Geometry check sheet. Reference: the model listing, model coordinates, mm. Face numbers are marked on the shaded views. A direction names the side the tool comes from. Round coordinates to 2 decimals unless told otherwise and drop trailing zeros. Write each loop counter-clockwise with the first axis right and the second up, starting at its lowest first coordinate (ties: lowest second). Pieces come first, ordered by that corner, then holes. Notation, with made-up numbers: (-17, -22.75) -> (0, -22.75) arc R11 ccw to (0, -4.75) -> close; hole circle Ø7 at (47, 38). An arc over 180 degrees is marked (long way). Use a Markdown table: item, result.
```python
from build123d import *

# Parameters (mm, degrees)
SKETCH1_R               = 13.85
BOSS_EXTRUDE1_DEPTH     = 63
CUT_EXTRUDE1_DEPTH      = 66.974578437
CUT_EXTRUDE1_DEPTH_BACK = 66.974578437


with BuildPart() as part:
    # Sketch1 → Boss-Extrude1 (new body)
    with BuildSketch(Plane.XY):
        Circle(SKETCH1_R)
    extrude(amount=BOSS_EXTRUDE1_DEPTH)

    # Sketch3 → Cut-Extrude1 (cut, two sides: drawn at the far end of the back side and taken through both)
    with BuildSketch(Plane(origin=(0, 0, 0), x_dir=(0, 0, -1), z_dir=(1, 0, 0)).offset(-CUT_EXTRUDE1_DEPTH_BACK)):
        with BuildLine():
            Line((0, 1.925), (-35.5, 1.925))
            ThreePointArc((-35.5, 1.925), (-37.267766953, 2.657233047), (-38, 4.425))
            Line((-38, 4.425), (-38, 13.85))
            Line((-38, 13.85), (0, 13.85))
            Line((0, 13.85), (0, 1.925))
        make_face()
        with BuildLine():
            Line((0, -1.925), (-45.5, -1.925))
            ThreePointArc((-45.5, -1.925), (-47.267766953, -2.657233047), (-48, -4.425))
            Line((-48, -4.425), (-48, -13.85))
            Line((-48, -13.85), (0, -13.85))
            Line((0, -13.85), (0, -1.925))
        make_face()
    extrude(amount=CUT_EXTRUDE1_DEPTH + CUT_EXTRUDE1_DEPTH_BACK, mode=Mode.SUBTRACT)


solid = part.part
```
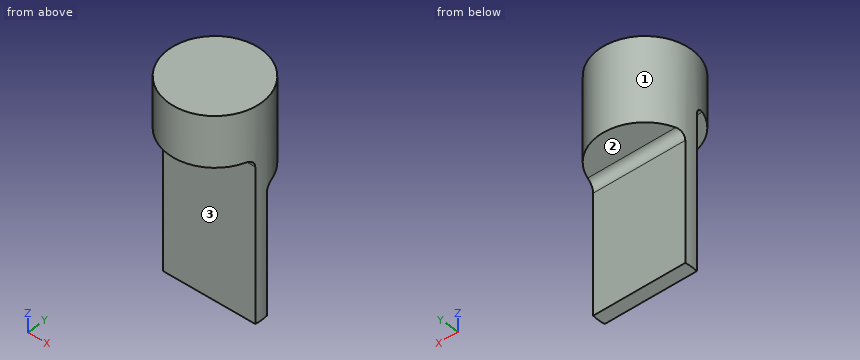
(1) Section check D-D on x = -9.75. Record the cut outline in (y, z) (3 decimals), plus the area to 3 significant figures.
A:
| item | result |
|---|---|
| outline | (-9.837, 48) -> (-4.425, 48) arc R2.5 cw to (-1.925, 45.5) -> (-1.925, 0) -> (1.925, 0) -> (1.925, 35.5) arc R2.5 cw to (4.425, 38) -> (9.837, 38) -> (9.837, 63) -> (-9.837, 63) -> close |
| area | 562 mm2 |
(2) Section check B-B on z = 27.5. Record the cut outline in (x, y) (3 decimals), plus the area to 3 significant figures.
A:
| item | result |
|---|---|
| outline | (-13.716, -1.925) -> (13.716, -1.925) arc R13.85 ccw to (13.716, 1.925) -> (-13.716, 1.925) arc R13.85 ccw to start |
| area | 106 mm2 |
(3) Thickness scan on line 1 (Y direction, x = 6, z = 30) (3 decimals); line 2 (Z direction, x = 3.25, y = 6.5); line 3 (Z direction, x = -6.75, y = -4.5). Record the ranges inside material, lowest first.
A:
| item | result |
|---|---|
| line 1 | y = -1.925 to 1.925 |
| line 2 | z = 38 to 63 |
| line 3 | z = 48 to 63 |
(4) Access from +Z, -Z, +X, -X, +Y, -Y to the whole of each face (thin tool, end or side, straight path). Record for the marked faces 1, 2 and 3.
A:
| item | result |
|---|---|
| face 1 | +Z, -Z |
| face 2 | -Z, +X, -X, +Y |
| face 3 | -Z, +X, -X, -Y |
(5) Section check A-A on x = 10.5. Record the cut outline in (y, z) (3 decimals), plus the area to 3 significant figures.
A:
| item | result |
|---|---|
| outline | (-9.032, 48) -> (-4.425, 48) arc R2.5 cw to (-1.925, 45.5) -> (-1.925, 0) -> (1.925, 0) -> (1.925, 35.5) arc R2.5 cw to (4.425, 38) -> (9.032, 38) -> (9.032, 63) -> (-9.032, 63) -> close |
| area | 530 mm2 |
(6) Section check C-C on y = 7.25. Record the cut outline in (x, z), plus the area to 3 significant figures.
A:
| item | result |
|---|---|
| outline | (-11.8, 38) -> (11.8, 38) -> (11.8, 63) -> (-11.8, 63) -> close |
| area | 590 mm2 |
(7) Gauge pin test, flat ends, axial feed: pin 1 Ø1.5 at (x, z) = (-0.5, 9.5) entering from -Y (3 decimals); pin 2 Ø1.5 at (x, y) = (-8, 9.5) entering from -Z; pin 3 Ø12 at (y, z) = (-10, 34.5) entering from +X; pin 4 Ø7.5 at (x, y) = (0, -7) entering from -Z. Record the tip position at first contact, or that the pin passes through.
A:
| item | result |
|---|---|
| pin 1 | stops at y = -1.925 |
| pin 2 | stops at z = 38 |
| pin 3 | passes through |
| pin 4 | stops at z = 47.71 |
